Autodesk Inventor part; units mm, degrees
ref_plane "YZ Plane" through (0, 0, 0) normal (1, 0, 0) x (0, 1, 0)
ref_plane "XZ Plane" through (0, 0, 0) normal (0, 1, 0) x (-1, 0, 0)
ref_plane "XY Plane" through (0, 0, 0) normal (0, 0, 1) x (1, 0, 0)
sketch "Sketch1" plane through (0, 0, 0) normal (0, 0, 1) x (1, 0, 0)
  circle A0 centre (0, 0) radius 9
  dimension "d0" = 18
extrude "Extrusion1" add sketch "Sketch1" along normal blind 4
sketch "Sketch2" plane through (0, 0, 4) normal (0, 0, 1) x (1, 0, 0)
  circle A0 centre (0, 0) radius 6
  circle A1 centre (0, 0) radius 3
  dimension "d3" = 12
  dimension "d4" = 6
extrude "Extrusion2" add sketch "Sketch2" along normal blind 40
sketch "Sketch4" plane through (0, 0, 4) normal (0, 0, 1) x (1, 0, 0)
  circle A0 centre (0, 0) radius 3
extrude "Extrusion3" add sketch "Sketch4" along normal blind 25.5
properties part number "Adaptateur_axes"
The listing builds one solid part. Answer for the finished solid, in the listing's coordinates (mm). A direction names the side the tool comes from. Coordinates: 2 decimals unless noted, no trailing zeros. Write each loop counter-clockwise with the first axis right and the second up, starting at its lowest first coordinate (ties: lowest second). Pieces come first, ordered by that corner, then holes. Notation, with made-up numbers: (40, 66.25) - (69, 66.25) arc R17 cw to (69, 87.25) - close; hole circle Ø2 at (-36, 14). An arc over 180 degrees is marked (long way). Return JSON: item names as keys, results as strings.
1. The part is cut by section B-B on z = 39. Determine the outline of the cut face in (x, y).
Final values:
{"outline": "circle Ø12 at (0, 0); hole circle Ø6 at (0, 0)"}
2. For a pull along Y with two mould halves and no side action, classify faces 1 (the face through (-6, 0, 24)), 2 (the face through (-3, 0, 37)), 3 (the face through (0, 0, 0)) as +Y half, -Y half, draft (parallel to the pull), parting line (faces both ways), or undercut.
Final values:
{"face 1": "parting line", "face 2": "undercut", "face 3": "draft"}
3. The part is cut by section D-D on z = 24. Determine the outline of the cut face in (x, y).
Final values:
{"outline": "circle Ø12 at (0, 0)"}
4. The part is cut by section A-A on y = 0. Determine the outline of the cut face in (x, z).
Final values:
{"outline": "(-9, 0) - (9, 0) - (9, 4) - (6, 4) - (6, 44) - (3, 44) - (3, 29.5) - (-3, 29.5) - (-3, 44) - (-6, 44) - (-6, 4) - (-9, 4) - close"}
5. Which of the six approach directions +Z, -Z, +X, -X, +Y, -Y give full straight-line access (tool end or side, diameter ignored) to faces 4 (the face through (-3, -1, 44)), 5 (the face through (2, -6, 4))?
Final values:
{"face 4": "+Z, +X, -X, +Y, -Y", "face 5": "+Z"}
6. Each of these flat-tipped pins is pushed along its axis until it touches: pin 1 Ø1 at (x, z) = (5, 36.5) entering from +Y; pin 2 Ø6 at (y, z) = (2, 24.5) entering from +X; pin 3 Ø4 at (y, z) = (5.5, 18.5) entering from -X. Where does it stop, or does it pass through?
Final values:
{"pin 1": "y = 3.97", "pin 2": "x = 6", "pin 3": "x = -4.87"}
7. Consider line 1 along Y through (x, z) = (0, 41.25); line 2 along Z through (x, y) = (5.5, -3.75); line 3 along Z through (x, y) = (1.5, -2). Determine where each line is inside the solid, lowest interval first.
Final values:
{"line 1": "-6 to -3, 3 to 6", "line 2": "0 to 4", "line 3": "0 to 29.5"}
